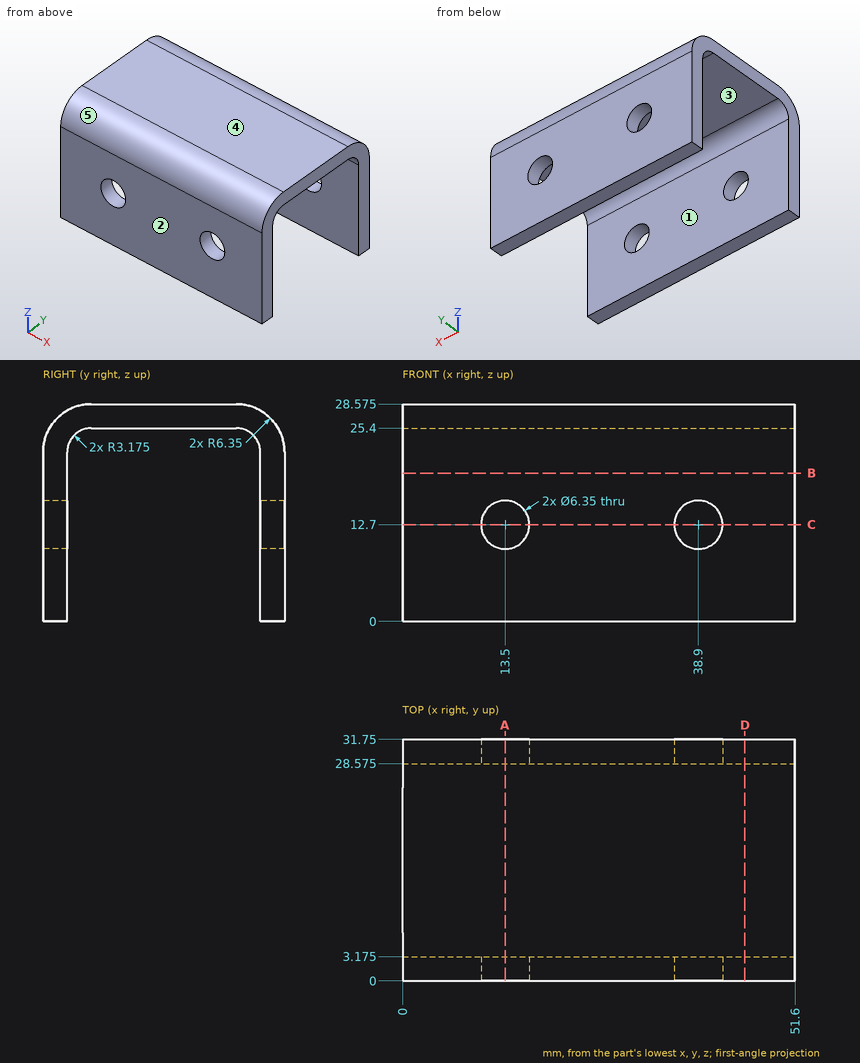
Input: dimensioned drawing with shaded views. Units: mm. Origin: part minimum x, y, z. A direction names the side the tool comes from. Give positions to 0.01 mm unless a question says otherwise; leave off trailing zeros. Loops run counter-clockwise (first coordinate to the right, second up) from the corner with the lowest first, then second, coordinate; pieces in that order, holes last. Notation, with made-up numbers: (-18.75, 82) - (-10.75, 82) arc R20 cw to (-10.75, 88) - close; hole circle Ø1 at (21, 0.5). An arc over 180 degrees is marked (long way). Answer as CSV lines item,"result". Start each with the question number.
(1) Section query C-C (z = 12.7). Output: boundary loops of the cut face in (x, y) (3 decimals).
(2) Ray query, line 1 along Y through (x, z) = (27.5, 16) (3 decimals); line 2 along Z through (x, y) = (6.5, 13.5) (3 decimals); line 3 along Z through (x, y) = (41.5, 30.5). Return the intervals inside material, ascending. Write a range as [from, to].
(3) Section query A-A (x = 13.5). Output: boundary loops of the cut face in (y, z) (3 decimals), and give its area (3 significant figures).
(4) Pin query (flat end, axial travel): P1, Ø5.5, axis at x = 17, y = 17.5, coming from the -Z side; P2, Ø10, axis at x = 42, y = 10.5, coming from the -Z side; P3, Ø7.5, axis at x = 13.5, z = 12.7, coming from the -Y side. Return the tip coordinate at first contact, or that it passes through.
(5) Reachability of the marked faces 1 and 2 from +Z, -Z, +X, -X, +Y, -Y: full face, straight path, thin tool, end or side. Return the list, or none.
(6) Section query D-D (x = 45). Output: boundary loops of the cut face in (y, z) (3 decimals).
(7) Section query B-B (z = 19.5). Output: boundary loops of the cut face in (x, y) (3 decimals), and give its area (3 significant figures).
(8) Mould query, pull axis Y, two halves, no side actions, for the marked faces 3, 4 and 5. Classes: +Y half, -Y half, draft (parallel to the pull), parting line (faces both ways), or undercut.
Worked answers:
1,outline,"(0, 0) - (10.325, 0) - (10.325, 3.175) - (0, 3.175) - close; (0, 28.575) - (10.325, 28.575) - (10.325, 31.75) - (0, 31.75) - close; (16.675, 0) - (35.725, 0) - (35.725, 3.175) - (16.675, 3.175) - close; (16.675, 28.575) - (35.725, 28.575) - (35.725, 31.75) - (16.675, 31.75) - close; (42.075, 0) - (51.6, 0) - (51.6, 3.175) - (42.075, 3.175) - close; (42.075, 28.575) - (51.6, 28.575) - (51.6, 31.75) - (42.075, 31.75) - close"
2,line 1,"y = [0, 3.175], [28.575, 31.75]"
2,line 2,"z = [25.4, 28.575]"
2,line 3,"z = [0, 10.88], [14.52, 26.01]"
3,outline,"(0, 0) - (3.175, 0) - (3.175, 9.525) - (0, 9.525) - close; (0, 15.875) - (3.175, 15.875) - (3.175, 22.225) arc R3.175 cw to (6.35, 25.4) - (25.4, 25.4) arc R3.175 cw to (28.575, 22.225) - (28.575, 15.875) - (31.75, 15.875) - (31.75, 22.225) arc R6.35 ccw to (25.4, 28.575) - (6.35, 28.575) arc R6.35 ccw to (0, 22.225) - close; (28.575, 0) - (31.75, 0) - (31.75, 9.525) - (28.575, 9.525) - close"
3,area,"209 mm^2"
4,P1,"stops at z = 25.4"
4,P2,"stops at z = 25.28"
4,P3,"stops at y = 0"
5,face 1,"-Z, +X, -X"
5,face 2,"+Z, -Z, +X, -X, -Y"
6,outline,"(0, 0) - (3.175, 0) - (3.175, 22.225) arc R3.175 cw to (6.35, 25.4) - (25.4, 25.4) arc R3.175 cw to (28.575, 22.225) - (28.575, 0) - (31.75, 0) - (31.75, 22.225) arc R6.35 ccw to (25.4, 28.575) - (6.35, 28.575) arc R6.35 ccw to (0, 22.225) - close"
7,outline,"(0, 0) - (51.6, 0) - (51.6, 3.175) - (0, 3.175) - close; (0, 28.575) - (51.6, 28.575) - (51.6, 31.75) - (0, 31.75) - close"
7,area,"328 mm^2"
8,face 3,"undercut"
8,face 4,"draft"
8,face 5,"-Y half"
